The listing builds one solid part. Answer for the finished solid, in the listing's coordinates (mm). Give positions to 0.01 mm unless a question says otherwise; leave off trailing zeros. Write each loop counter-clockwise with the first axis right and the second up, starting at its lowest first coordinate (ties: lowest second). Pieces come first, ordered by that corner, then holes. Notation, with made-up numbers: (-34.75, -37) - (15.25, -37) arc R19 cw to (15.25, -23) - close; hole circle Ø8 at (-16.5, 4). An arc over 180 degrees is marked (long way). One line per item, written item: value. Start each with the question number.
from build123d import *

# Parameters (mm, degrees)
F0_W     = 440
F0_H     = 230
F1_DEPTH = 3
F2_W     = 300
F2_H     = 33
F2_R     = 1.35
F2_R_2   = 3.1
F3_DEPTH = 3.001
F4_R     = 10
F5_R     = 5


with BuildPart() as f1:
    # F0 (on Top) → F1 (new body)
    with BuildSketch(Plane.XY):
        with Locations((220, 115)):
            Rectangle(F0_W, F0_H)
    extrude(amount=F1_DEPTH)

    # F2 (on face) → F3 (cut, through all)
    with BuildSketch(Plane.XY.offset(3)):
        with Locations((195, 153.5)):
            Rectangle(F2_W, F2_H)
        with Locations((40, 153.5)):
            Circle(F2_R)
        with Locations((75, 174)):
            Circle(F2_R)
        with Locations((75, 133)):
            Circle(F2_R)
        with Locations((135, 174)):
            Circle(F2_R)
        with Locations((135, 133)):
            Circle(F2_R)
        with Locations((195, 174)):
            Circle(F2_R)
        with Locations((195, 133)):
            Circle(F2_R)
        with Locations((255, 174)):
            Circle(F2_R)
        with Locations((255, 133)):
            Circle(F2_R)
        with Locations((315, 174)):
            Circle(F2_R)
        with Locations((315, 133)):
            Circle(F2_R)
        with Locations((350, 153.5)):
            Circle(F2_R)
        with Locations((7, 7)):
            Circle(F2_R_2)
        with Locations((7, 115)):
            Circle(F2_R_2)
        with Locations((147, 7)):
            Circle(F2_R_2)
        with Locations((287, 7)):
            Circle(F2_R_2)
        with Locations((427, 7)):
            Circle(F2_R_2)
        with Locations((427, 115)):
            Circle(F2_R_2)
        with Locations((7, 223)):
            Circle(F2_R_2)
        with Locations((147, 223)):
            Circle(F2_R_2)
        with Locations((287, 223)):
            Circle(F2_R_2)
        with Locations((427, 223)):
            Circle(F2_R_2)
    extrude(amount=-F3_DEPTH, mode=Mode.SUBTRACT)

    # F4
    f4_edges = [f1.edges().sort_by_distance(p)[0] for p in [
        (440, 0, 1.5),
        (0, 0, 1.5),
        (440, 230, 1.5),
        (0, 230, 1.5),
    ]]
    fillet(f4_edges, radius=F4_R)

    # F5
    f5_edges = [f1.edges().sort_by_distance(p)[0] for p in [
        (45, 137, 1.5),
        (45, 170, 1.5),
        (345, 170, 1.5),
        (345, 137, 1.5),
    ]]
    fillet(f5_edges, radius=F5_R)


solid = f1.part
Item 1: Find section A-A on x = 220.5. Determine the outline of the cut face in (y, z), plus the area to 3 significant figures.
Item 2: Straight lines are drawn through the part: line 1 along X through (y, z) = (174, 1.95); line 2 along Y through (x, z) = (255, 1.15); line 3 along Y through (x, z) = (287, 0.7). For each, find the intervals that lie inside material, in ascending order.
Item 3: Find section B-B on z = 2.3. Give the number of separate pieces and of enclosed holes in the cut face, plus the area to 3 significant figures.
Values:
1. outline: (0, 0) - (137, 0) - (137, 3) - (0, 3) - close; (170, 0) - (230, 0) - (230, 3) - (170, 3) - close
1. area: 591 mm^2
2. line 1: 0 to 73.65, 76.35 to 133.65, 136.35 to 193.65, 196.35 to 253.65, 256.35 to 313.65, 316.35 to 440
2. line 2: 0 to 131.65, 134.35 to 137, 170 to 172.65, 175.35 to 230
2. line 3: 0 to 3.9, 10.1 to 137, 170 to 219.9, 226.1 to 230
3. separate pieces: 1
3. enclosed holes: 23
3. area: 90,900 mm^2
